The model under review builds one solid part; all positions refer to its coordinate system, in mm. Face numbers are marked on the shaded views. A direction names the side the tool comes from. Coordinates: 2 decimals unless noted, no trailing zeros. Order: outer loops, then holes, each group sorted by start corner. A loop starts at its lowest first (then second) coordinate and runs counter-clockwise, first axis right, second up. Notation, with made-up numbers: (20, 1.25) -> (47, 1.25) arc R6 ccw to (47, 8.25) -> close; hole circle Ø5 at (21.5, -15). An arc over 180 degrees is marked (long way). Use one line per item in the form item = value.
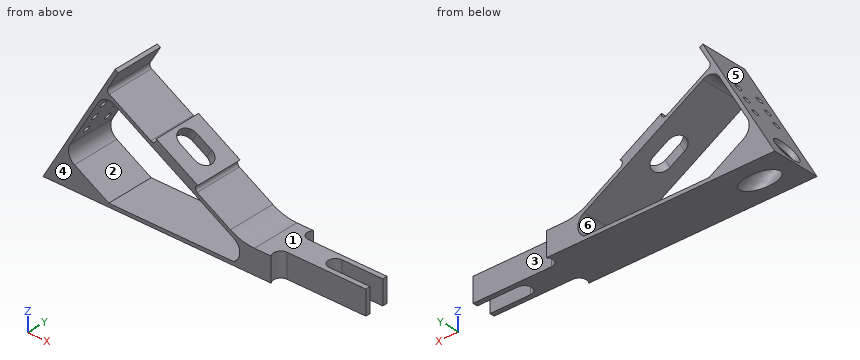
from build123d import *

# Parameters (mm, degrees)
F0_W     = 35
F0_H     = 10
F1_DEPTH = 10
F3_DEPTH = 4
F4_R     = 1.395
F5_DEPTH = 1.5
F4_R_2   = 5.5
F4_R_3   = 4.25
F6_DEPTH = 2
F7_DEPTH = 112.584302492
F9_DEPTH = 10.001


with BuildPart() as f1:
    # F0 (on Front) → F1 (new body, symmetric)
    with BuildSketch(Plane.XZ):
        with BuildLine():
            Line((30, 51.9615242271), (0, 0))
            Line((0, 0), (95, 0))
            Line((95, 0), (95, 10))
            Line((95, 10), (88.0384757729, 10))
            ThreePointArc((88.0384757729, 10), (82.8620948709, 10.6814834742), (78.0384757729, 12.6794919243))
            Line((78.0384757729, 12.6794919243), (64.1755840358, 20.6832362005))
            ThreePointArc((64.1755840358, 20.6832362005), (63.4335436954, 22.1365974171), (64.4573381993, 23.4073167043))
            Line((64.4573381993, 23.4073167043), (47.1368301236, 33.4073167043))
            ThreePointArc((47.1368301236, 33.4073167043), (46.5482521918, 31.8853250121), (44.918584287, 31.8012701892))
            Line((44.918584287, 31.8012701892), (27.5980762114, 41.8012701892))
            ThreePointArc((27.5980762114, 41.8012701892), (26.8991874719, 42.7120797272), (27.0490381057, 43.8503082949))
            Line((27.0490381057, 43.8503082949), (31.2990381057, 51.2115242271))
            Line((31.2990381057, 51.2115242271), (30, 51.9615242271))
        make_face()
        with BuildLine():
            Line((11.2990381057, 16.5705080757), (23.0490381057, 36.9221050646))
            ThreePointArc((23.0490381057, 36.9221050646), (26.0850698991, 39.2517341961), (29.8791651246, 38.7522320835))
            Line((29.8791651246, 38.7522320835), (79.4019237886, 10.1602540378))
            ThreePointArc((79.4019237886, 10.1602540378), (81.9019237886, 5.8301270189), (79.4019237886, 1.5))
            Line((79.4019237886, 1.5), (27.4019237886, 1.5))
            Line((27.4019237886, 1.5), (13.1291651246, 9.7403810568))
            ThreePointArc((13.1291651246, 9.7403810568), (10.7995359932, 12.7764128502), (11.2990381057, 16.5705080757))
        make_face(mode=Mode.SUBTRACT)
        with Locations((112.5, 5)):
            Rectangle(F0_W, F0_H)
    extrude(amount=F1_DEPTH, both=True)

    # F2 (on face) → F3 (cut)
    with BuildSketch(Plane(origin=(26.25, 0, 45.4663336987), x_dir=(0.8660254038, 0, -0.5), z_dir=(0.5, 0, 0.8660254038))):
        with BuildLine():
            ThreePointArc((29.5, 4), (25.5, 0), (29.5, -4))
            Line((29.5, -4), (36.5, -4))
            ThreePointArc((36.5, -4), (40.5, 0), (36.5, 4))
            Line((36.5, 4), (29.5, 4))
        make_face()
    extrude(amount=-F3_DEPTH, mode=Mode.SUBTRACT)

    # F4 (on face) → F5 (cut)
    with BuildSketch(Plane(origin=(0, 0, 0), x_dir=(0, -1, 0), z_dir=(-0.8660254038, 0, 0.5))):
        with Locations((-5, 39)):
            Circle(F4_R)
        with Locations((-5, 32)):
            Circle(F4_R)
        with Locations((5, 25)):
            Circle(F4_R)
        with Locations((5, 32)):
            Circle(F4_R)
        with Locations((5, 39)):
            Circle(F4_R)
        with Locations((-5, 25)):
            Circle(F4_R)
    extrude(amount=-F5_DEPTH, mode=Mode.SUBTRACT)

    # F4 (on face) → F6 (cut)
    with BuildSketch(Plane(origin=(0, 0, 0), x_dir=(0, -1, 0), z_dir=(-0.8660254038, 0, 0.5))):
        with Locations((0, 7.5)):
            Circle(F4_R_2)
        with Locations((0, 7.5)):
            Circle(F4_R_3, mode=Mode.SUBTRACT)
    extrude(amount=-F6_DEPTH, mode=Mode.SUBTRACT)

    # F7 (cut, through all): a face of the model
    f7_faces = [f1.faces().sort_by_distance(p)[0] for p in [
        (3.75, 0, 6.4951905284),
    ]]
    extrude(f7_faces, amount=-F7_DEPTH, mode=Mode.SUBTRACT)

    # F8 (on face) → F9 (cut, through all)
    with BuildSketch(Plane.XY.offset(10)):
        with BuildLine():
            Line((130, -10), (130, -5))
            Line((130, -5), (97.2360679775, -5))
            ThreePointArc((97.2360679775, -5), (94.49745519, -6.7752551286), (95, -10))
            Line((95, -10), (130, -10))
        make_face()
        with BuildLine():
            Line((130, -3), (130, 3))
            Line((130, 3), (113, 3))
            ThreePointArc((113, 3), (110, 0), (113, -3))
            Line((113, -3), (130, -3))
        make_face()
        with BuildLine():
            Line((97.2360679775, 5), (130, 5))
            Line((130, 5), (130, 10))
            Line((130, 10), (95, 10))
            ThreePointArc((95, 10), (94.49745519, 6.7752551286), (97.2360679775, 5))
        make_face()
    extrude(amount=-F9_DEPTH, mode=Mode.SUBTRACT)


solid = f1.part
Item 1: We need section C-C (x = 86.5). Write out the cut boundary in (y, z), plus the area to 3 significant figures.
Results found:
outline = (-10, 0) -> (10, 0) -> (10, 10.06) -> (-10, 10.06) -> close
area = 201 mm²
Item 2: To check wall thickness, follow L1, parallel to Y at x = 56, z = 24; L2, parallel to Z at x = 50.5, y = 2.5; L3, parallel to Y at x = 11, z = 5.5. State the ranges of each line that lie inside material, in increasing order. Write a range as from..to.
Results found:
L1 = -10..-4, 4..10
L2 = 0..1.5
L3 = -10..-3.23, 3.23..10
Item 3: Tool access review of the marked faces 1, 2 and 3: name each direction out of +Z, -Z, +X, -X, +Y, -Y from which nothing blocks a thin tool from reaching the whole face with its end or side.
Results found:
face_1 = +Z, +X, +Y, -Y
face_2 = +Y, -Y
face_3 = +Z, -Z, +X, +Y
Item 4: Draft analysis for pull direction X (two halves, no side actions). For the marked faces 4, 5 and 6, state which applies: released by +X, released by -X, zero draft, split by the parting line, or undercut.
Results found:
face_4 = zero draft
face_5 = released by -X
face_6 = undercut
Item 5: Clearance check with flat-ended pins moving along their axes: pin 1 (8 mm diameter, centred on x = 122, z = 6, fed in from -Y); pin 2 (3 mm diameter, centred on x = 116.5, z = 3, fed in from +Y); pin 3 (4 mm diameter, centred on x = 36.5, y = -3, fed in from +Z). State where each tip first meets the part, or that it passes through.
Results found:
pin_1 = -5
pin_2 = 5
pin_3 = 37.82
Item 6: We need section A-A (x = 70). Write out the cut boundary in (y, z), plus the area to 3 significant figures.
Results found:
outline = (-10, 0) -> (10, 0) -> (10, 1.5) -> (-10, 1.5) -> close; (-10, 15.59) -> (10, 15.59) -> (10, 17.32) -> (-10, 17.32) -> close
area = 64.6 mm²
Item 7: We need section B-B (x = 102.5). Write out the cut boundary in (y, z).
Results found:
outline = (-5, 0) -> (5, 0) -> (5, 10) -> (-5, 10) -> close
